Geometry check sheet. Reference: the model listing, model coordinates, mm. Face numbers are marked on the shaded views. Coordinates: 2 decimals unless noted, no trailing zeros. Write each loop counter-clockwise with the first axis right and the second up, starting at its lowest first coordinate (ties: lowest second). Pieces come first, ordered by that corner, then holes. Notation, with made-up numbers: (59, 74) -> (65, 74) arc R14 cw to (65, 82) -> close; hole circle Ø1 at (-37, -16). An arc over 180 degrees is marked (long way). Answer as CSV lines item,"result".
```python
from build123d import *

# Parameters (mm, degrees)
SKETCH1_W           = 67
SKETCH1_H           = 56.5
SKETCH1_R           = 2.5
BOSS_EXTRUDE1_DEPTH = 3
BOSS_EXTRUDE2_DEPTH = 67
BOSS_EXTRUDE3_DEPTH = 4
BOSS_EXTRUDE4_DEPTH = 4
BOSS_EXTRUDE5_REACH = 79.461
SKETCH6_W           = 1.5
SKETCH6_H           = 1


with BuildPart() as part:
    # Sketch1 → Boss-Extrude1 (new body)
    with BuildSketch(Plane.XY):
        Rectangle(SKETCH1_W, SKETCH1_H)
        with Locations((-28.25, 23.5)):
            Circle(SKETCH1_R, mode=Mode.SUBTRACT)
        with Locations((-18.75, 23.5)):
            Circle(SKETCH1_R, mode=Mode.SUBTRACT)
        with Locations((-9.25, 23.5)):
            Circle(SKETCH1_R, mode=Mode.SUBTRACT)
        with Locations((0.25, 23.5)):
            Circle(SKETCH1_R, mode=Mode.SUBTRACT)
        with Locations((9.75, 23.5)):
            Circle(SKETCH1_R, mode=Mode.SUBTRACT)
        with Locations((19.25, 23.5)):
            Circle(SKETCH1_R, mode=Mode.SUBTRACT)
        with Locations((28.75, 23.5)):
            Circle(SKETCH1_R, mode=Mode.SUBTRACT)
        with Locations((-18.75, 14)):
            Circle(SKETCH1_R, mode=Mode.SUBTRACT)
        with Locations((-9.25, 14)):
            Circle(SKETCH1_R, mode=Mode.SUBTRACT)
        with Locations((0.25, 14)):
            Circle(SKETCH1_R, mode=Mode.SUBTRACT)
        with Locations((9.75, 14)):
            Circle(SKETCH1_R, mode=Mode.SUBTRACT)
        with Locations((19.25, 14)):
            Circle(SKETCH1_R, mode=Mode.SUBTRACT)
        with Locations((28.75, 14)):
            Circle(SKETCH1_R, mode=Mode.SUBTRACT)
        with Locations((-18.75, 4.5)):
            Circle(SKETCH1_R, mode=Mode.SUBTRACT)
        with Locations((-9.25, 4.5)):
            Circle(SKETCH1_R, mode=Mode.SUBTRACT)
        with Locations((0.25, 4.5)):
            Circle(SKETCH1_R, mode=Mode.SUBTRACT)
        with Locations((9.75, 4.5)):
            Circle(SKETCH1_R, mode=Mode.SUBTRACT)
        with Locations((19.25, 4.5)):
            Circle(SKETCH1_R, mode=Mode.SUBTRACT)
        with Locations((28.75, 4.5)):
            Circle(SKETCH1_R, mode=Mode.SUBTRACT)
        with Locations((-18.75, -5)):
            Circle(SKETCH1_R, mode=Mode.SUBTRACT)
        with Locations((-9.25, -5)):
            Circle(SKETCH1_R, mode=Mode.SUBTRACT)
        with Locations((0.25, -5)):
            Circle(SKETCH1_R, mode=Mode.SUBTRACT)
        with Locations((9.75, -5)):
            Circle(SKETCH1_R, mode=Mode.SUBTRACT)
        with Locations((19.25, -5)):
            Circle(SKETCH1_R, mode=Mode.SUBTRACT)
        with Locations((28.75, -5)):
            Circle(SKETCH1_R, mode=Mode.SUBTRACT)
        with Locations((-18.75, -14.5)):
            Circle(SKETCH1_R, mode=Mode.SUBTRACT)
        with Locations((-9.25, -14.5)):
            Circle(SKETCH1_R, mode=Mode.SUBTRACT)
        with Locations((0.25, -14.5)):
            Circle(SKETCH1_R, mode=Mode.SUBTRACT)
        with Locations((9.75, -14.5)):
            Circle(SKETCH1_R, mode=Mode.SUBTRACT)
        with Locations((19.25, -14.5)):
            Circle(SKETCH1_R, mode=Mode.SUBTRACT)
        with Locations((28.75, -14.5)):
            Circle(SKETCH1_R, mode=Mode.SUBTRACT)
        with Locations((-18.75, -24)):
            Circle(SKETCH1_R, mode=Mode.SUBTRACT)
        with Locations((-9.25, -24)):
            Circle(SKETCH1_R, mode=Mode.SUBTRACT)
        with Locations((0.25, -24)):
            Circle(SKETCH1_R, mode=Mode.SUBTRACT)
        with Locations((9.75, -24)):
            Circle(SKETCH1_R, mode=Mode.SUBTRACT)
        with Locations((19.25, -24)):
            Circle(SKETCH1_R, mode=Mode.SUBTRACT)
        with Locations((28.75, -24)):
            Circle(SKETCH1_R, mode=Mode.SUBTRACT)
        with Locations((-28.25, 14)):
            Circle(SKETCH1_R, mode=Mode.SUBTRACT)
        with Locations((-28.25, 4.5)):
            Circle(SKETCH1_R, mode=Mode.SUBTRACT)
        with Locations((-28.25, -5)):
            Circle(SKETCH1_R, mode=Mode.SUBTRACT)
        with Locations((-28.25, -14.5)):
            Circle(SKETCH1_R, mode=Mode.SUBTRACT)
        with Locations((-28.25, -24)):
            Circle(SKETCH1_R, mode=Mode.SUBTRACT)
    extrude(amount=BOSS_EXTRUDE1_DEPTH)

    # Sketch2 → Boss-Extrude2 (add)
    with BuildSketch(Plane(origin=(33.5, 0, 0), x_dir=(0, 0, -1), z_dir=(1, 0, 0))):
        Polygon((0, -28.25), (-3, -28.25), (-3, -35.25), (5.4, -35.25), (5.4, -28.25), (3.4, -28.25), (3.4, -33.25), (2, -33.25), (2, -28.25), align=None)
    extrude(amount=-BOSS_EXTRUDE2_DEPTH)

    # Sketch3 → Boss-Extrude3 (add)
    with BuildSketch(Plane.ZY.offset(33.5)):
        Polygon((-5.4, -28.25), (-23.7, -35.25), (21.3, -35.25), (3, -28.25), align=None)
    extrude(amount=BOSS_EXTRUDE3_DEPTH)

    # Sketch4 → Boss-Extrude4 (add)
    with BuildSketch(Plane(origin=(33.5, 0, 0), x_dir=(0, 0, -1), z_dir=(1, 0, 0))):
        Polygon((5.4, -28.25), (23.7, -35.25), (-21.3, -35.25), (-3, -28.25), align=None)
    extrude(amount=BOSS_EXTRUDE4_DEPTH)

    # Boss-Extrude5: up to this face of the body (flat: up to its plane)
    boss_extrude5_end = Plane(part.part.faces().sort_by_distance((0, 28.25, 1.5))[0])
    # Sketch6 → Boss-Extrude5 (add, up to the picked face)
    with BuildSketch(Plane.XZ.offset(35.25), mode=Mode.PRIVATE) as boss_extrude5_sk1:
        Polygon((-33.5, 3), (-33.5, 3.5), (-33.5, 4.5), (-37.5, 4.5), (-37.5, 0), (-33.5, 0), align=None)
    boss_extrude5_tool1 = split(extrude(boss_extrude5_sk1.sketch, amount=-BOSS_EXTRUDE5_REACH, mode=Mode.PRIVATE), bisect_by=boss_extrude5_end, keep=Keep.BOTH, mode=Mode.PRIVATE)
    # Sketch6 → Boss-Extrude5 (add, up to the picked face)
    with BuildSketch(Plane.XZ.offset(35.25), mode=Mode.PRIVATE) as boss_extrude5_sk2:
        with Locations((-32.75, 4)):
            Rectangle(SKETCH6_W, SKETCH6_H)
    boss_extrude5_tool2 = split(extrude(boss_extrude5_sk2.sketch, amount=-BOSS_EXTRUDE5_REACH, mode=Mode.PRIVATE), bisect_by=boss_extrude5_end, keep=Keep.BOTH, mode=Mode.PRIVATE)
    # Sketch6 → Boss-Extrude5 (add, up to the picked face)
    with BuildSketch(Plane.XZ.offset(35.25), mode=Mode.PRIVATE) as boss_extrude5_sk3:
        Polygon((33.5, 4.5), (33.5, 3.5), (33.5, 3), (33.5, 0), (37.5, 0), (37.5, 4.5), align=None)
    boss_extrude5_tool3 = split(extrude(boss_extrude5_sk3.sketch, amount=-BOSS_EXTRUDE5_REACH, mode=Mode.PRIVATE), bisect_by=boss_extrude5_end, keep=Keep.BOTH, mode=Mode.PRIVATE)
    # Sketch6 → Boss-Extrude5 (add, up to the picked face)
    with BuildSketch(Plane.XZ.offset(35.25), mode=Mode.PRIVATE) as boss_extrude5_sk4:
        with Locations((32.75, 4)):
            Rectangle(SKETCH6_W, SKETCH6_H)
    boss_extrude5_tool4 = split(extrude(boss_extrude5_sk4.sketch, amount=-BOSS_EXTRUDE5_REACH, mode=Mode.PRIVATE), bisect_by=boss_extrude5_end, keep=Keep.BOTH, mode=Mode.PRIVATE)
    add(boss_extrude5_tool1.solids().sort_by(Axis((-35.5, -35.25, 2.25), (0, 1, 0)))[0])
    add(boss_extrude5_tool2.solids().sort_by(Axis((-32.75, -35.25, 4), (0, 1, 0)))[0])
    add(boss_extrude5_tool3.solids().sort_by(Axis((35.5, -35.25, 2.25), (0, 1, 0)))[0])
    add(boss_extrude5_tool4.solids().sort_by(Axis((32.75, -35.25, 4), (0, 1, 0)))[0])


solid = part.part
```
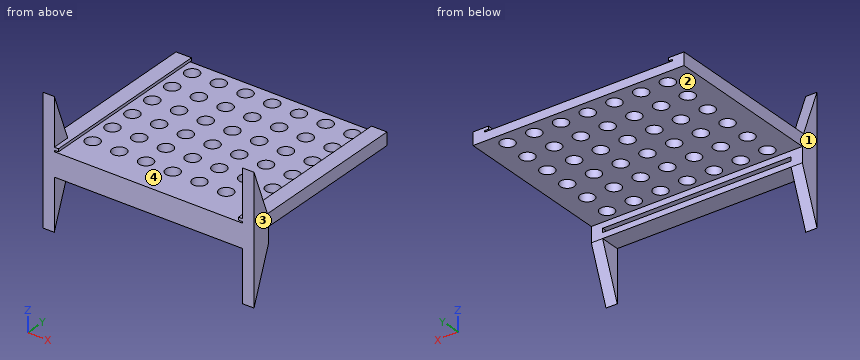
Item 1: Release check for a two-part mould opening along X. For the marked faces 1, 2, 3 and 4 record: +X half, -X half, draft (parallel to the pull), parting line (faces both ways), or undercut.
Responses:
face 1,"-X half"
face 2,"draft"
face 3,"+X half"
face 4,"undercut"
Item 2: Cross-section at C-C, the plane x = 4. Record the cut outline in (y, z), plus the area to 3 significant figures.
Responses:
outline,"(-35.25, -5.4) -> (-28.25, -5.4) -> (-28.25, -3.4) -> (-33.25, -3.4) -> (-33.25, -2) -> (-28.25, -2) -> (-28.25, 0) -> (28.25, 0) -> (28.25, 3) -> (-35.25, 3) -> close"
area,"221 mm2"
Item 3: Cross-section at B-B, the plane z = 11. Record the cut outline in (x, y), plus the area to 3 significant figures.
Responses:
outline,"(-37.5, -35.25) -> (-33.5, -35.25) -> (-33.5, -31.31) -> (-37.5, -31.31) -> close; (33.5, -35.25) -> (37.5, -35.25) -> (37.5, -31.31) -> (33.5, -31.31) -> close"
area,"31.5 mm2"
Item 4: Depth check by flat-ended pin: pin 1 Ø8 at (x, y) = (-18.75, -24) entering from +Z; pin 2 Ø1 at (x, y) = (-5.5, -6) entering from -Z; pin 3 Ø12 at (x, z) = (-8.5, 12) entering from -Y; pin 4 Ø5.5 at (x, y) = (-5, -31.5) entering from -Z. Enter the tip coordinate at first touch or a pass-through.
Responses:
pin 1,"stops at z = 3"
pin 2,"stops at z = 0"
pin 3,"passes through"
pin 4,"stops at z = -5.4"
Item 5: Cross-section at D-D, the plane y = 8.5. Record the cut outline in (x, z).
Responses:
outline,"(-37.5, 0) -> (37.5, 0) -> (37.5, 4.5) -> (32, 4.5) -> (32, 3.5) -> (33.5, 3.5) -> (33.5, 3) -> (-33.5, 3) -> (-33.5, 3.5) -> (-32, 3.5) -> (-32, 4.5) -> (-37.5, 4.5) -> close"
Item 6: Cross-section at A-A, the plane x = 28.75. Count the separate pieces of the cut face and the enclosed holes in it, plus the area to 3 significant figures.
Responses:
separate pieces,"7"
enclosed holes,"0"
area,"131 mm2"
Item 7: Thickness scan on probe 1 along X at (y, z) = (8, 4); probe 2 along Z at (x, y) = (1, -29); probe 3 along Z at (x, y) = (27, -8.5). Record the ranges inside material, lowest first.
Responses:
probe 1,"x = -37.5 to -32, 32 to 37.5"
probe 2,"z = -5.4 to -3.4, -2 to 3"
probe 3,"z = 0 to 3"
